Here's the drawing with two shaded views (mm, measured from the low corner). I have some questions. Give positions to 0.01 mm unless a question says otherwise; leave off trailing zeros. Order: outer loops, then holes, each group sorted by start corner. A loop starts at its lowest first (then second) coordinate and runs counter-clockwise, first axis right, second up. Notation, with made-up numbers: M 78,17 L 97,17 A27 ccw 97,38 Z; hole C 43.25,-18 d1. An arc over 180 degrees is marked long. Write each question's results on one line, items separated by ' | '.
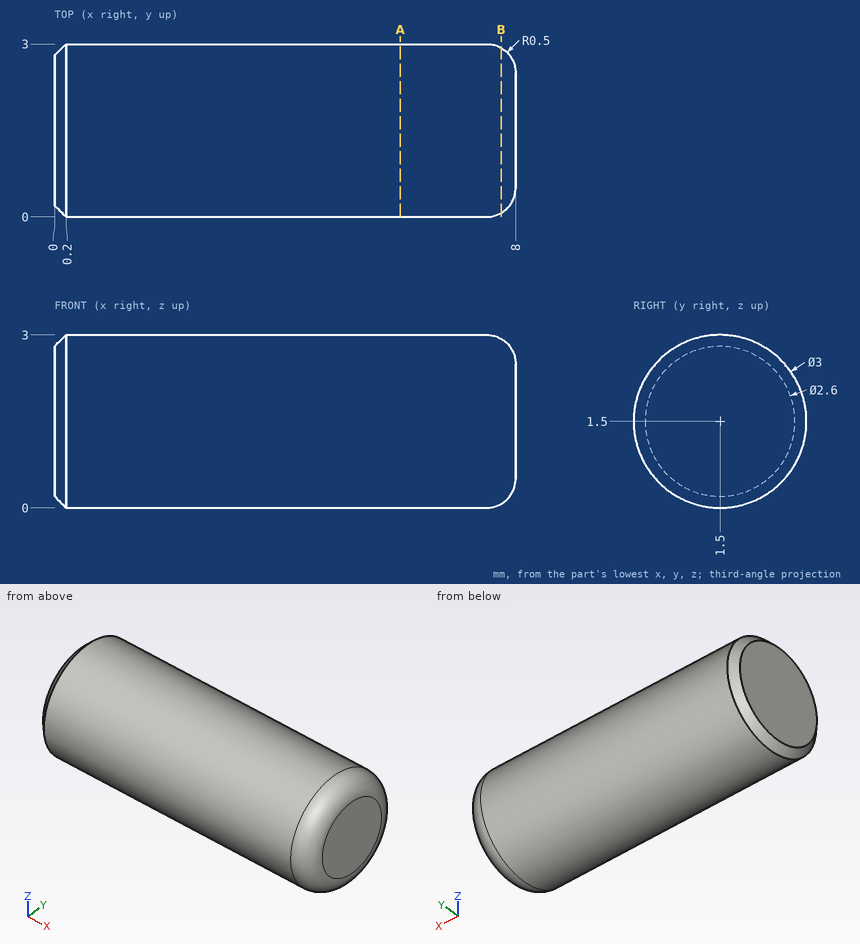
(1) I need wall thicknesses on L1, parallel to X at y = 1.9, z = 2.65; L2, parallel to Y at x = 1.25, z = 1.05; L3, parallel to Z at x = 2.5, y = 0.45. Which ranges of each line are inside material? Lowest first, please. Write a range as from..to.
Data:
L1: x = 0..7.95 | L2: y = 0.07..2.93 | L3: z = 0.43..2.57
(2) Imagine slicing it at B-B, the plane x = 7.75. Write out the boundary of the cut face in (y, z), plus the area to 3 significant figures.
Data:
outline: C 1.5,1.5 d2.87 | area: 6.45 mm2
(3) Imagine slicing it at A-A, the plane x = 6. Write out the boundary of the cut face in (y, z), plus the area to 3 significant figures.
Data:
outline: C 1.5,1.5 d3 | area: 7.07 mm2
